```python
from build123d import *

# Parameters (mm, degrees)
SKIZZE4_R                       = 2.5
SCHNITT_LINEAR_AUSTRAGEN1_DEPTH = 20.5


with BuildPart() as part:
    # Skizze3 → Rotation1 (revolve)
    with BuildSketch(Plane(origin=(0, 0, 0), x_dir=(1, 0, 0), z_dir=(0, 1, 0))):
        Polygon((0, 0), (32, 0), (32, 6), (9, 6), (9, 9), (0, 9), align=None)
    revolve(axis=Axis((0, 0, 0), (1, 0, 0)))

    # Skizze4 → Schnitt-Linear austragen1 (cut)
    with BuildSketch(Plane.ZY):
        Circle(SKIZZE4_R)
    extrude(amount=-SCHNITT_LINEAR_AUSTRAGEN1_DEPTH, mode=Mode.SUBTRACT)


solid = part.part
```
Input: part model. Units: mm. Frame: model coordinates. A direction names the side the tool comes from. Round coordinates to 2 decimals unless told otherwise and drop trailing zeros. Loops run counter-clockwise (first coordinate to the right, second up) from the corner with the lowest first, then second, coordinate; pieces in that order, holes last. Notation, with made-up numbers: M 42,31.25 L 71,31.25 A13 cw 71,40.25 Z; hole C -20,-23.5 d10. An arc over 180 degrees is marked long. Answer in a Markdown table with one row per item. Add a question column.
1. Ray query, probe 1 along Y at (x, z) = (4, 0); probe 2 along Y at (x, z) = (14.5, 0); probe 3 along X at (y, z) = (-7.75, 4). Return the intervals inside material, ascending.
2. Mould query, pull axis Z, two halves, no side actions, for faces 1 (the face through (10.11, -2.44, -0.54)), 2 (the face through (32, 0, 0)), 3 (the face through (4.437, 8.923, 1.172)). Classes: released by +Z, released by -Z, zero draft, split by the parting line, or undercut.
3. Section D-D (x = 24.5). Output: boundary loops of the cut face in (y, z), and give its area (3 significant figures).
4. Set-up query: faces 4 (the face through (20.5, 0, 0)), 5 (the face through (0, -2, -2)), 6 (the face through (9, -6, 2)). Return all of +Z, -Z, +X, -X, +Y, -Y with unobstructed straight access to the full face (end or side cutting, diameter ignored); none if empty.
5. Section A-A (z = 0). Output: boundary loops of the cut face in (x, y), and give its area (4 significant figures).
6. Contact query for flat-ended pins moving along their axis: pin 1 (1 mm diameter, centred on x = 6, z = 3, fed in from +Y); pin 2 (3 mm diameter, centred on x = 26, y = -3, fed in from -Z); pin 3 (1 mm diameter, centred on x = 13, z = 0.5, fed in from -Y). Output: stop coordinate, or through.
7. Section B-B (x = 3). Output: boundary loops of the cut face in (y, z).
Values follow:
| question | item | result |
|---|---|---|
| 1 | probe 1 | -9 to -2.5, 2.5 to 9 |
| 1 | probe 2 | -6 to -2.5, 2.5 to 6 |
| 1 | probe 3 | 0 to 9 |
| 2 | face 1 | undercut |
| 2 | face 2 | zero draft |
| 2 | face 3 | split by the parting line |
| 3 | outline | C 0,0 d12 |
| 3 | area | 113 mm^2 |
| 4 | face 4 | -X |
| 4 | face 5 | +Z, -Z, -X, +Y, -Y |
| 4 | face 6 | +X |
| 5 | outline | M 0,-9 L 9,-9 L 9,-6 L 32,-6 L 32,6 L 9,6 L 9,9 L 0,9 L 0,2.5 L 20.5,2.5 L 20.5,-2.5 L 0,-2.5 Z |
| 5 | area | 335.5 mm^2 |
| 6 | pin 1 | y = 8.65 |
| 6 | pin 2 | z = -5.81 |
| 6 | pin 3 | y = -6 |
| 7 | outline | C 0,0 d18; hole C 0,0 d5 |
